Build history of the part. All positions in model axes, mm. Face numbers are marked on the shaded views. A direction names the side the tool comes from. Coordinates: 2 decimals unless noted, no trailing zeros. Order: outer loops, then holes, each group sorted by start corner. A loop starts at its lowest first (then second) coordinate and runs counter-clockwise, first axis right, second up. Notation, with made-up numbers: (53, 28.25) - (84, 28.25) arc R22 ccw to (84, 64.25) - close; hole circle Ø8 at (-23, 29). An arc over 180 degrees is marked (long way). Write each question's results on one line, items separated by ' | '. Start each with the question number.
Solid Edge part; units mm, degrees
sketch "Sketch1" plane through (0, 0, 0) normal (0, -1, 0) x (1, 0, 0)
  line L0 (0, 36) -> (-80, 36)
  line L1 (-80, 36) -> (-80, 24)
  line L2 (-80, 24) -> (-12, 24)
  line L3 (-12, 24) -> (-12, -24)
  line L4 (-80, -24) -> (-12, -24)
  line L5 (-80, -36) -> (-80, -24)
  line L6 (0, -36) -> (-80, -36)
  line L7 (0, -6) -> (0, -36)
  line L8 (80, -6) -> (0, -6)
  line L9 (80, 6) -> (80, -6)
  line L10 (0, 6) -> (80, 6)
  line L11 (0, 6) -> (0, 36)
extrude "Protrusion1" add sketch "Sketch1" against normal blind 60
sketch "Sketch2" plane through (-40, 30, 36) normal (0, 0, 1) x (1, 0, 0)
  circle A0 centre (90, 0) radius 10
  circle A1 centre (-10, 0) radius 10
extrude "ExtrudedCutout_1" cut sketch "Sketch2" against normal blind 72
fillet "Round_2" radius 30 1 edges at (80, 60, 0)
fillet "Round_3" radius 30 5 edges at (80, 0, 0) (-80, 0, 30) (-80, 0, -30) (-80, 60, -30) (-80, 60, 30)
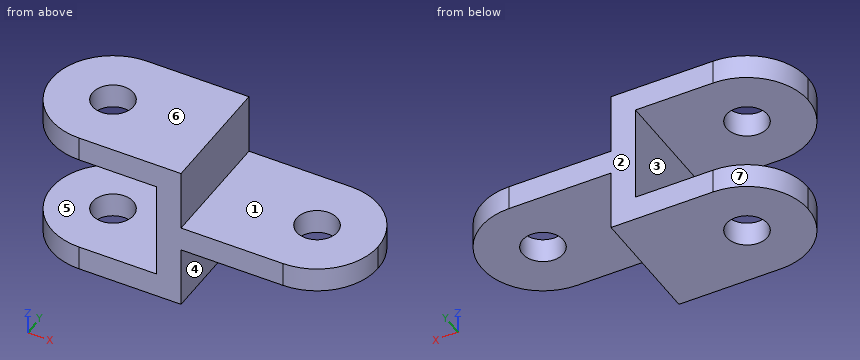
Item 1: Slice it at B-B (y = 38.5). Write the cut outline in (x, z).
Item 2: Slice it at A-A (x = -42). Write the cut outline in (y, z).
Item 3: Probe probe 1 along Z at (x, y) = (-27.5, 5); probe 2 along Y at (x, z) = (-50, 31.5); probe 3 along Z at (x, y) = (24, 23.5). List the from-to ranges inside material, lowest first.
Item 4: Pull direction Z, two halves, no side cores. Call the marked faces 5, 6 and 7: released by +Z, released by -Z, zero draft, split by the parting line, or undercut.
Item 5: Slice it at C-C (x = 48.5). Write the cut outline in (y, z).
Item 6: Which spindle directions (+Z, -Z, +X, -X, +Y, -Y) get a long thin tool onto all of the face, cutting with end or side? Do the marked faces 1, 2, 3 and 4. Say none if no direction does.
Item 7: Slice it at D-D (z = 15). Write the cut outline in (x, y), then the cut area to 3 significant figures.
Item 8: Flat gauge pins, fed straight in: P1, Ø15, axis at y = 27, z = -19, coming from the +X side; P2, Ø4, axis at y = 45, z = 2.5, coming from the -X side; P3, Ø6, axis at x = 30, y = 11.5, coming from the -Z side. Where does each tip first touch, or does it go through?
Resolved:
1) outline: (-78.77, -36) - (-55.27, -36) - (-55.27, -24) - (-78.77, -24) - close; (-78.77, 24) - (-55.27, 24) - (-55.27, 36) - (-78.77, 36) - close; (-44.73, -36) - (0, -36) - (0, -6) - (44.73, -6) - (44.73, 6) - (0, 6) - (0, 36) - (-44.73, 36) - (-44.73, 24) - (-12, 24) - (-12, -24) - (-44.73, -24) - close; (55.27, -6) - (78.77, -6) - (78.77, 6) - (55.27, 6) - close
2) outline: (0, -36) - (24, -36) - (24, -24) - (0, -24) - close; (0, 24) - (24, 24) - (24, 36) - (0, 36) - close; (36, -36) - (60, -36) - (60, -24) - (36, -24) - close; (36, 24) - (60, 24) - (60, 36) - (36, 36) - close
3) probe 1: -36 to -24, 24 to 36 | probe 2: 0 to 20, 40 to 60 | probe 3: -6 to 6
4) face 5: undercut | face 6: released by +Z | face 7: zero draft
5) outline: (0, -6) - (20.11, -6) - (20.11, 6) - (0, 6) - close; (39.89, -6) - (60, -6) - (60, 6) - (39.89, 6) - close
6) face 1: +Z, +X, +Y, -Y | face 2: +Z, -Z, +X, -X, +Y | face 3: -X, +Y, -Y | face 4: -Z, +X, +Y, -Y
7) outline: (-12, 0) - (0, 0) - (0, 60) - (-12, 60) - close | area: 720 mm^2
8) P1: x = 0 | P2: x = -12 | P3: z = -6
